from build123d import *

# Parameters (mm, degrees)
F1_ANGLE       = 90
F2_W           = 35
F2_H           = 35
F2_R           = 7.5
F3_ANGLE       = 5
F4_ANGLE_START = 270
F4_ANGLE       = 5
F5_W           = 10
F5_H           = 109.1421356237
F6_ANGLE_START = 280
F6_ANGLE       = 70


with BuildPart() as f1:
    # F0 (on Front) → F1 (revolve)
    with BuildSketch(Plane.XZ):
        Polygon((0, -86.7003262881), (0, 63.2996737119), (-42.5, 63.2996737119), (-42.5, 3.2996737119), (-32.5, 3.2996737119), (-32.5, 48.2996737119), (-10, 48.2996737119), (-10, -90.8424619118), (24.4289321881, -125.2713940999), (31.5, -118.2003262881), align=None)
    revolve(axis=Axis((-319.5, 0, -5.3764432669), (0, 0, -1)), revolution_arc=F1_ANGLE)

    # F2 (on face) → F3 (revolve)
    with BuildSketch(Plane(origin=(-319.5, 0, 0), x_dir=(0, -1, 0), z_dir=(-1, 0, 0))):
        with Locations((337, 30.7996737119)):
            Rectangle(F2_W, F2_H)
        with Locations((337, 30.7996737119)):
            Circle(F2_R, mode=Mode.SUBTRACT)
        with Locations((337, -54.2003262881)):
            Rectangle(F2_W, F2_H)
        with Locations((337, -54.2003262881)):
            Circle(F2_R, mode=Mode.SUBTRACT)
    revolve(axis=Axis((-319.5, 0, 7.2890669107), (0, 0, 1)), revolution_arc=F3_ANGLE)

    # F2 (on face) → F4 (revolve)
    with BuildSketch(Plane(origin=(-319.5, 0, 0), x_dir=(0, -1, 0), z_dir=(-1, 0, 0)), mode=Mode.PRIVATE) as f4_sk:
        with Locations((337, 30.7996737119)):
            Rectangle(F2_W, F2_H)
        with Locations((337, 30.7996737119)):
            Circle(F2_R, mode=Mode.SUBTRACT)
        with Locations((337, -54.2003262881)):
            Rectangle(F2_W, F2_H)
        with Locations((337, -54.2003262881)):
            Circle(F2_R, mode=Mode.SUBTRACT)
    revolve(f4_sk.sketch.rotate(Axis((-319.5, 0, 63.2996737119), (0, 0, -1)), F4_ANGLE_START), axis=Axis((-319.5, 0, 63.2996737119), (0, 0, -1)), revolution_arc=F4_ANGLE)

    # F5 (on Front) → F6 (revolve, cut)
    with BuildSketch(Plane.XZ, mode=Mode.PRIVATE) as f6_sk:
        with Locations((-5, -6.2713940999)):
            Rectangle(F5_W, F5_H)
    revolve(f6_sk.sketch.rotate(Axis((-319.5, 0, -29.9057289958), (0, 0, 1)), F6_ANGLE_START), axis=Axis((-319.5, 0, -29.9057289958), (0, 0, 1)), revolution_arc=F6_ANGLE, mode=Mode.SUBTRACT)


solid = f1.part
Here's how the part is built. I have some questions about the finished solid (model axes, mm). A direction names the side the tool comes from. Round coordinates to 2 decimals unless told otherwise and drop trailing zeros. Order: outer loops, then holes, each group sorted by start corner. A loop starts at its lowest first (then second) coordinate and runs counter-clockwise, first axis right, second up. Notation, with made-up numbers: M -22,8.25 L -7,8.25 A25 cw -7,42.25 Z; hole C 9,-6 d5. An arc over 180 degrees is marked long. One line per question, with ' | ' between items.
1) Imagine slicing it at B-B, the plane z = -19. Write out the boundary of the cut face in (x, y), plus the area to 3 significant figures.
Checked values:
outline: M -319.5,-319.5 A319.5 ccw -264.02,-314.65 L -265.76,-304.8 A309.5 cw -319.5,-309.5 Z; M -14.7,-53.74 L -4.85,-55.48 A319.5 ccw 0,0 L -10,0 A309.5 cw Z | area: 1,100 mm²
2) On a 3-axis mill with a long thin cutter (end or side, diameter ignored), from which of +Z, -Z, +X, -X, +Y, -Y can I reach the whole of each face in a straight line? I mean faces 1 (the flat face through (-290.15, -335.47, 38.82)), 2 (the flat face through (-264.9, -309.65, -5.51)), 3 (the flat face through (-122, -197, 3.3)), 4 (the flat face through (8.225, -28.672, 31.045)), 5 (the cylindrical face through (34.67, -15.25, 31.04)). Say none if no direction works.
Checked values:
face 1: +Z, +X | face 2: +X | face 3: -Z, -X, +Y | face 4: +Z, -Y | face 5: +Z, -Z, +X, -Y
3) I need wall thicknesses on line 1 (Z direction, x = -191, y = -287.5); line 2 (Z direction, x = -16, y = -128); line 3 (Z direction, x = -70, y = -230). Which ranges of each line are inside material? Lowest first, please.
Checked values:
line 1: z = -96.25 to -60.84, 48.3 to 63.3 | line 2: z = -110.73 to -96.59 | line 3: z = -120.68 to -106.54
4) I'm going to push flat-ended pins straight in: pin 1 Ø1.5 at (y, z) = (-266, -101) entering from -X; pin 2 Ø12 at (x, z) = (-20, -79) entering from -Y; pin 3 Ø4 at (x, z) = (-36, -83) entering from -Y; pin 4 Ø15.5 at (x, y) = (21, -18) entering from -Z. Where does each tip first touch, or does it pass through?
Checked values:
pin 1: stops at x = -144 | pin 2: stops at y = -126.25 | pin 3: stops at y = -151.12 | pin 4: stops at z = -125.27
5) We'd pull the mould along X, two halves only. Please class faces 6 (the conical face through (-96.72, -217.94, -93)), 7 (the flat face through (-9.85, -54.6, -5.51)), 8 (the flat face through (17, -16, 48.3)): released by +X, released by -X, zero draft, split by the parting line, or undercut.
Checked values:
face 6: released by -X | face 7: undercut | face 8: zero draft
6) Imagine slicing it at A-A, the plane z = 8. Write out the boundary of the cut face in (x, y), plus the area to 3 significant figures.
Checked values:
outline: M -319.5,-319.5 A319.5 ccw -264.02,-314.65 L -265.76,-304.8 A309.5 cw -319.5,-309.5 Z; M -319.5,-287 A287 ccw -32.5,0 L -42.5,0 A277 cw -319.5,-277 Z; M -14.7,-53.74 L -4.85,-55.48 A319.5 ccw 0,0 L -10,0 A309.5 cw Z | area: 5,530 mm²
7) Imagine slicing it at C-C, the plane z = -66. Write out the boundary of the cut face in (x, y), plus the area to 3 significant figures.
Checked values:
outline: M -319.5,-354.5 A354.5 ccw -288.6,-353.15 L -291.65,-318.28 A319.5 ccw -1.22,-27.85 L 33.65,-30.9 A354.5 ccw 35,0 L -10,0 A309.5 cw -319.5,-309.5 Z | area: 7,000 mm²
